The drawing under review shows one solid part. Ordinate dimensions are in mm from its lowest x, y, z. Give positions to 0.01 mm unless a question says otherwise; leave off trailing zeros. Order: outer loops, then holes, each group sorted by start corner. A loop starts at its lowest first (then second) coordinate and runs counter-clockwise, first axis right, second up. Notation, with made-up numbers: (7, 22) -> (33, 22) arc R15 cw to (33, 51) -> close; hole circle Ø6 at (1.25, 6.5). An arc over 180 degrees is marked (long way). Use a Markdown table: item, result. Add a question column.
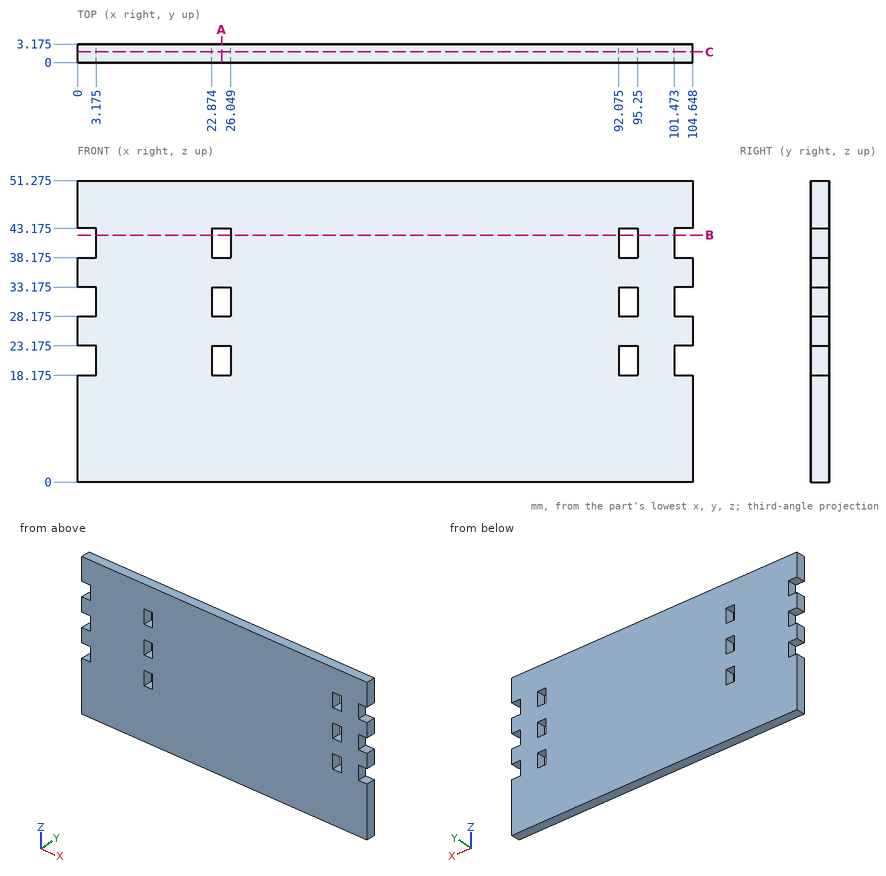
1) Add section B-B (z = 42). Give the boundary of the cut face in (x, y) (3 decimals), then the cut area to 3 significant figures.
2) Insertion check: pin 1 (1.6 mm diameter, centred on y = 1, z = 31, fed in from -X) (3 decimals); pin 2 (1.6 mm diameter, centred on y = 1.5, z = 21.5, fed in from +X). Each pin has a flat end and moves straight along its axis. Give the tip position at first contact, or say it passes through.
3) Add section C-C (y = 1.85). Give the number of separate pieces and of enclosed holes in the cut face, then the cut area to 3 significant figures.
4) For L1, parallel to Z at x = 94.5, y = 0.45 (3 decimals); L2, parallel to X at y = 2.95, z = 29 (3 decimals), list the stretches that pass through material, from the lowest coordinate up. Write a range as [from, to].
5) Add section A-A (x = 24.5). Give the boundary of the cut face in (y, z) (3 decimals).
Worked answers:
| question | item | result |
|---|---|---|
| 1 | outline | (3.175, 0) -> (22.874, 0) -> (22.874, 3.175) -> (3.175, 3.175) -> close; (26.049, 0) -> (92.075, 0) -> (92.075, 3.175) -> (26.049, 3.175) -> close; (95.25, 0) -> (101.473, 0) -> (101.473, 3.175) -> (95.25, 3.175) -> close |
| 1 | area | 292 mm^2 |
| 2 | pin 1 | x = 3.175 |
| 2 | pin 2 | x = 101.47 |
| 3 | separate pieces | 1 |
| 3 | enclosed holes | 6 |
| 3 | area | 5,180 mm^2 |
| 4 | L1 | [0, 18.175], [23.175, 28.175], [33.175, 38.175], [43.175, 51.275] |
| 4 | L2 | [3.175, 22.874], [26.049, 92.075], [95.25, 101.473] |
| 5 | outline | (0, 0) -> (3.175, 0) -> (3.175, 18.175) -> (0, 18.175) -> close; (0, 23.175) -> (3.175, 23.175) -> (3.175, 28.175) -> (0, 28.175) -> close; (0, 33.175) -> (3.175, 33.175) -> (3.175, 38.175) -> (0, 38.175) -> close; (0, 43.175) -> (3.175, 43.175) -> (3.175, 51.275) -> (0, 51.275) -> close |
